```python
from build123d import *

# Parameters (mm, degrees)
CHANFREIN2_SIZE  = 1
CHANFREIN2_SIZE2 = 2.144506921


with BuildPart() as part:
    # Esquisse1 → Révolution16 (revolve)
    with BuildSketch(Plane.XY, mode=Mode.PRIVATE) as r_volution16_sk:
        Polygon((7, 3), (10, 3), (10, 1.5), (13.5, 1.5), (13.5, 1), (21.5, 1), (21.5, 0), (0, 0), (0, 2.5), (7, 2.5), align=None)
    revolve(r_volution16_sk.sketch.rotate(Axis((0, 0, 0), (1, 0, 0)), 180), axis=Axis((0, 0, 0), (1, 0, 0)))

    # Chanfrein2
    chanfrein2_edges = [part.edges().sort_by_distance(p)[0] for p in [
        (10, 3, 0),
    ]]
    chanfrein2_side = [part.faces().sort_by_distance(p)[0] for p in [
        (10, 2.915147186, 0),
    ]]
    chamfer(chanfrein2_edges, length=CHANFREIN2_SIZE, length2=CHANFREIN2_SIZE2, reference=chanfrein2_side[0])


solid = part.part
```
Geometry: final body of the model. Coordinates: model frame, mm. A direction names the side the tool comes from. Round coordinates to 2 decimals unless told otherwise and drop trailing zeros. Order: outer loops, then holes, each group sorted by start corner. A loop starts at its lowest first (then second) coordinate and runs counter-clockwise, first axis right, second up. Notation, with made-up numbers: (66.5, -10) - (123.5, -10) arc R32 ccw to (123.5, 29) - close; hole circle Ø1 at (-39, 82). An arc over 180 degrees is marked (long way). Write item = value, one per line. Start each with the question number.
Q1. Cut plane D-D on x = 11. Return the cut outline in (y, z), and give its area (3 significant figures).
Q2. Cut plane C-C on x = 14. Return the cut outline in (y, z).
Q3. Access query for faces 1 (the cylindrical face through (18, 0, 1)), 2 (the flat face through (0, 0, 0)), 3 (the cylindrical face through (3.5, 2.5, -0.1)). Directions: +Z, -Z, +X, -X, +Y, -Y. A direction counts if a zero-diameter tool reaches every point of the face in a straight line with its end or side. Return the directions, or none.
Q4. Ray query, line 1 (X direction, y = -1.4, z = 0.15); line 2 (X direction, y = -1.8, z = -0.8); line 3 (Z direction, x = 6.5, y = 1.35). Return the intervals inside material, ascending. Write a range as from..to.
Q5. Pin query (flat end, axial travel): pin 1 (1 mm diameter, centred on x = 7.5, y = 1, fed in from -Z); pin 2 (2 mm diameter, centred on x = 3, z = 0, fed in from +Y). Return the tip coordinate at first contact, or that it passes through.
Q6. Cut plane A-A on y = 0. Return the cut outline in (x, z), and give its area (3 significant figures).
Outcome:
q1.outline = circle Ø3 at (0, 0)
q1.area = 7.07 mm^2
q2.outline = circle Ø2 at (0, 0)
q3.face_1 = +X
q3.face_2 = +Z, -Z, -X, +Y, -Y
q3.face_3 = -X
q4.line_1 = 0..13.5
q4.line_2 = 0..10
q4.line_3 = -2.1..2.1
q5.pin_1 = -2.96
q5.pin_2 = 2.5
q6.outline = (0, -2.5) - (7, -2.5) - (7, -3) - (7.86, -3) - (10, -2) - (10, -1.5) - (13.5, -1.5) - (13.5, -1) - (21.5, -1) - (21.5, 1) - (13.5, 1) - (13.5, 1.5) - (10, 1.5) - (10, 2) - (7.86, 3) - (7, 3) - (7, 2.5) - (0, 2.5) - close
q6.area = 77.4 mm^2
